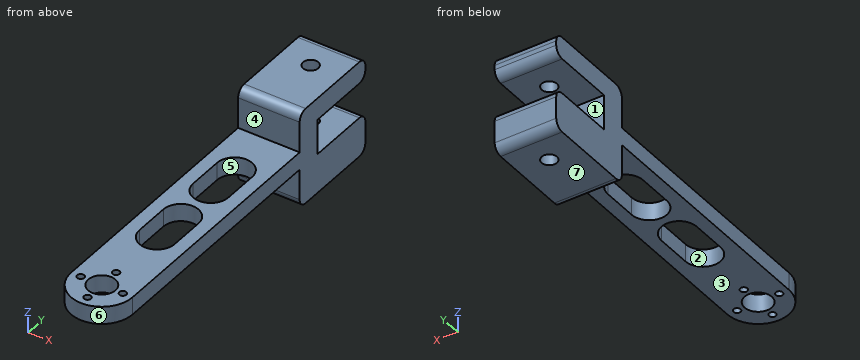
```python
from build123d import *

# Parameters (mm, degrees)
BOSS_EXTRUDE1_DEPTH = 5
BOSS_EXTRUDE2_DEPTH = 17.5
CUT_EXTRUDE1_DEPTH  = 35
SKETCH13_R          = 4.35
CUT_EXTRUDE7_DEPTH  = 129.671092325
CUT_EXTRUDE2_DEPTH  = 10
CUT_EXTRUDE3_DEPTH  = 10
SKETCH9_R           = 7.75
SKETCH9_R_2         = 2
CUT_EXTRUDE4_DEPTH  = 121.778723292


with BuildPart() as part:
    # Sketch2 → Boss-Extrude1 (new, symmetric)
    with BuildSketch(Plane.XY):
        with BuildLine():
            Line((17.5, 97.5), (-17.5, 97.5))
            Line((-17.5, 97.5), (-17.5, -97.5))
            ThreePointArc((-17.5, -97.5), (0, -115), (17.5, -97.5))
            Line((17.5, -97.5), (17.5, 97.5))
        make_face()
    extrude(amount=BOSS_EXTRUDE1_DEPTH, both=True)

    # Sketch3 → Boss-Extrude2 (add, symmetric)
    with BuildSketch(Plane(origin=(0, 0, 0), x_dir=(0, 0, -1), z_dir=(1, 0, 0))):
        with BuildLine():
            Line((-22.5, 97.5), (22.5, 97.5))
            ThreePointArc((22.5, 97.5), (26.035533906, 96.035533906), (27.5, 92.5))
            Line((27.5, 92.5), (27.5, 47.5))
            ThreePointArc((27.5, 47.5), (26.035533906, 43.964466094), (22.5, 42.5))
            Line((22.5, 42.5), (-22.5, 42.5))
            ThreePointArc((-22.5, 42.5), (-26.035533906, 43.964466094), (-27.5, 47.5))
            Line((-27.5, 47.5), (-27.5, 92.5))
            ThreePointArc((-27.5, 92.5), (-26.035533906, 96.035533906), (-22.5, 97.5))
        make_face()
    extrude(amount=BOSS_EXTRUDE2_DEPTH, both=True)

    # Sketch4 → Cut-Extrude1 (cut)
    with BuildSketch(Plane.ZY.offset(17.5)):
        with BuildLine():
            Line((-5, 92.5), (-5, 57.5))
            Line((-5, 57.5), (15, 57.5))
            Line((15, 57.5), (15, 92.5))
            ThreePointArc((15, 92.5), (16.464466094, 96.035533906), (20, 97.5))
            Line((20, 97.5), (-10, 97.5))
            ThreePointArc((-10, 97.5), (-6.464466094, 96.035533906), (-5, 92.5))
        make_face()
    extrude(amount=-CUT_EXTRUDE1_DEPTH, mode=Mode.SUBTRACT)

    # Sketch13 → Cut-Extrude7 (cut, through all)
    with BuildSketch(Plane(origin=(0, 0, -27.5), x_dir=(-1, 0, 0), z_dir=(0, 0, -1))):
        with Locations(Location((0, 77.5, 0), (0, 0, 90))):
            Circle(SKETCH13_R)
    extrude(amount=-CUT_EXTRUDE7_DEPTH, mode=Mode.SUBTRACT)

    # Sketch5 → Cut-Extrude2 (cut)
    with BuildSketch(Plane.XY.offset(5)):
        with BuildLine():
            Line((10, 13.756181567), (10, -6.243818433))
            ThreePointArc((10, -6.243818433), (0, -16.243818433), (-10, -6.243818433))
            Line((-10, -6.243818433), (-10, 13.756181567))
            ThreePointArc((-10, 13.756181567), (0, 23.756181567), (10, 13.756181567))
        make_face()
        with BuildLine():
            Line((10, -31.243818433), (10, -51.243818433))
            ThreePointArc((10, -51.243818433), (0, -61.243818433), (-10, -51.243818433))
            Line((-10, -51.243818433), (-10, -31.243818433))
            ThreePointArc((-10, -31.243818433), (0, -21.243818433), (10, -31.243818433))
        make_face()
    cut_extrude2 = extrude(amount=-CUT_EXTRUDE2_DEPTH, mode=Mode.SUBTRACT)

    # Mirror1: Cut-Extrude2 across plane
    add(cut_extrude2.mirror(Plane.XY), mode=Mode.SUBTRACT)

    # Sketch8 → Cut-Extrude3 (cut)
    with BuildSketch(Plane.XY.offset(5)):
        with BuildLine():
            Line((5, 13.756181567), (5, -6.243818433))
            ThreePointArc((5, -6.243818433), (0, -11.243818433), (-5, -6.243818433))
            Line((-5, -6.243818433), (-5, 13.756181567))
            ThreePointArc((-5, 13.756181567), (0, 18.756181567), (5, 13.756181567))
        make_face()
        with BuildLine():
            Line((-5, -31.243818433), (-5, -51.243818433))
            ThreePointArc((-5, -51.243818433), (0, -56.243818433), (5, -51.243818433))
            Line((5, -51.243818433), (5, -31.243818433))
            ThreePointArc((5, -31.243818433), (0, -26.243818433), (-5, -31.243818433))
        make_face()
    extrude(amount=-CUT_EXTRUDE3_DEPTH, mode=Mode.SUBTRACT)

    # Sketch9 → Cut-Extrude4 (cut, through all)
    with BuildSketch(Plane(origin=(0, 0, -5), x_dir=(-1, 0, 0), z_dir=(0, 0, -1))):
        with Locations((0, -97.5)):
            Circle(SKETCH9_R)
        with Locations((12, -97.5)):
            Circle(SKETCH9_R_2)
        with Locations((0, -109.5)):
            Circle(SKETCH9_R_2)
        with Locations((-12, -97.5)):
            Circle(SKETCH9_R_2)
        with Locations((0, -85.5)):
            Circle(SKETCH9_R_2)
    extrude(amount=-CUT_EXTRUDE4_DEPTH, mode=Mode.SUBTRACT)


solid = part.part
```
Here's how the part is built. I have some questions about the finished solid (model axes, mm). Face numbers are marked on the shaded views. A direction names the side the tool comes from. Coordinates: 2 decimals unless noted, no trailing zeros. Order: outer loops, then holes, each group sorted by start corner. A loop starts at its lowest first (then second) coordinate and runs counter-clockwise, first axis right, second up.
Item 1: If we section it at D-D, the plane x = -12: List the corners of the cut face in (y, z) for me, then the cut area to 3 significant figures.
Response values:
outline: (-110.24, -5) - (-99.5, -5) - (-99.5, 5) - (-110.24, 5) - close; (-95.5, -5) - (42.5, -5) - (42.5, -22.5) arc R5 ccw to (47.5, -27.5) - (92.5, -27.5) arc R5 ccw to (97.5, -22.5) - (97.5, -10) arc R5 ccw to (92.5, -5) - (57.5, -5) - (57.5, 15) - (92.5, 15) arc R5 ccw to (97.5, 20) - (97.5, 22.5) arc R5 ccw to (92.5, 27.5) - (47.5, 27.5) arc R5 ccw to (42.5, 22.5) - (42.5, 5) - (-95.5, 5) - close
area: 3,680 mm2
Item 2: If we section it at A-A, the plane y = 77.5: List the corners of the cut face in (x, z) for me, then the cut area to 4 significant figures.
Response values:
outline: (-17.5, -27.5) - (-4.35, -27.5) - (-4.35, -5) - (-17.5, -5) - close; (-17.5, 15) - (-4.35, 15) - (-4.35, 27.5) - (-17.5, 27.5) - close; (4.35, -27.5) - (17.5, -27.5) - (17.5, -5) - (4.35, -5) - close; (4.35, 15) - (17.5, 15) - (17.5, 27.5) - (4.35, 27.5) - close
area: 920.5 mm2
Item 3: If we section it at C-C, the plane z = -20: List the corners of the cut face in (x, y) for me.
Response values:
outline: (-17.5, 42.5) - (17.5, 42.5) - (17.5, 97.5) - (-17.5, 97.5) - close; hole circle Ø8.7 at (0, 77.5)
Item 4: Thinking about a two-plate mould opening in X: for the marked faces 5, 6 and 7, which applies, pulls with the +X half, pulls with the -X half, needs draft (parallel to the pull), parting line crosses it, or undercut?
Response values:
face 5: undercut
face 6: parting line crosses it
face 7: needs draft
Item 5: I'm going to push flat-ended pins straight in: pin 1 Ø9 at (x, z) = (-8, -13.5) entering from -Y; pin 2 Ø6 at (x, z) = (-12.5, -5.5) entering from -Y; pin 3 Ø5 at (x, z) = (-2, -4.5) entering from +Y; pin 4 Ø3 at (x, y) = (0, -85.5) entering from -Z. Where does each tip first touch, or does it pass through?
Response values:
pin 1: stops at y = 42.5
pin 2: stops at y = -112.17
pin 3: stops at y = 96.5
pin 4: passes through
Item 6: I need wall thicknesses on probe 1 along Y at (x, z) = (0, 1.25); probe 2 along X at (y, z) = (77, -11); probe 3 along Z at (x, y) = (-12.5, -39). Which ranges of each line are inside material? Lowest first, please.
Response values:
probe 1: y = -115 to -111.5, -107.5 to -105.25, -89.75 to -87.5, -83.5 to -61.24, -21.24 to -16.24, 23.76 to 57.5
probe 2: x = -17.5 to -4.32, 4.32 to 17.5
probe 3: z = -5 to 5
Item 7: If we section it at B-B, the plane y = 1.5: List the corners of the cut face in (x, z) for me.
Response values:
outline: (-17.5, -5) - (-10, -5) - (-10, 5) - (-17.5, 5) - close; (10, -5) - (17.5, -5) - (17.5, 5) - (10, 5) - close
Item 8: Which directions (+Z, -Z, +X, -X, +Y, -Y) give clear straight access to the entire face, cutting with the end or side of a thin tool? Please do the marked faces 1, 2, 3 and 4.
Response values:
face 1: +X, -X, +Y
face 2: +Z, -Z
face 3: -Z, +X, -X, -Y
face 4: +Z, +X, -X, -Y
